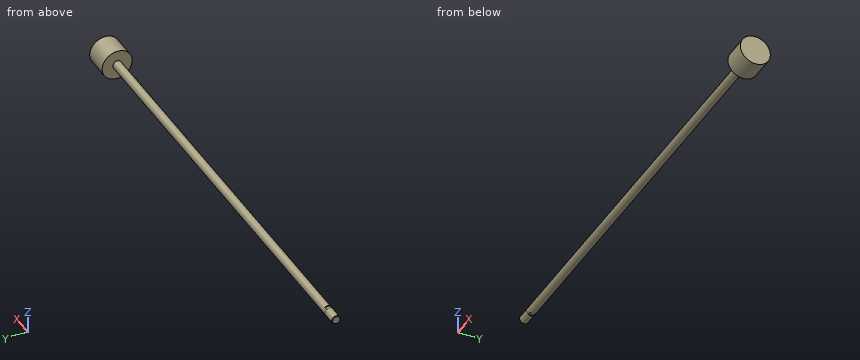
Autodesk Inventor part; units mm, degrees
ref_plane "rod_cp_XY" through (0, 0, 0) normal (1, 0, 0) x (0, 0, -1)
ref_plane "rod_cp_YZ" through (0, 0, 0) normal (0, 0, -1) x (0, 1, 0)
ref_plane "rod_cp_ZX" through (0, 0, 0) normal (0, 1, 0) x (1, 0, 0)
sketch "Sketch_1" plane through (0, 0, 0) normal (0, 0, 1) x (1, 0, 0)
  line L0 (393.5984, 0) -> (-3.175, 0)
  line L1 (-3.175, 0) -> (-3.175, 3.9624)
  line L2 (-3.175, 3.9624) -> (371.475, 3.9624)
  line L3 (371.475, 3.9624) -> (371.475, 13.5572)
  line L4 (371.475, 13.5572) -> (393.5984, 13.5572)
  line L5 (393.5984, 13.5572) -> (393.5984, 0)
  line L6 (393.5984, 0) -> (-3.175, 0)
revolve "Revolution1" add sketch "Sketch_1" angle 360 about axis through (393.5984, 0, 0) along (1, 0, 0)
sketch "Sketch_3" plane through (0, 0, 0) normal (0, 0, 1) x (1, 0, 0)
  line L0 (-3.175, 0) -> (-15.875, 0)
  line L1 (-15.875, 0) -> (-15.875, 3.3388)
  line L2 (-15.875, 3.3388) -> (-15.2451, 3.9688)
  line L3 (-15.2451, 3.9688) -> (-3.175, 3.9688)
  line L4 (-3.175, 3.9688) -> (-3.175, 0)
  line L5 (-3.175, 0) -> (-15.875, 0)
revolve "Revolution2" add sketch "Sketch_3" angle 360 about axis through (-3.175, 0, 0) along (1, 0, 0)
thread "Thread1"
sketch "Sketch_10" plane through (-3.175, 0, 0) normal (1, 0, 0) x (0, 0, -1)
  line L0 (-7.9248, 7.9248) -> (-7.9248, -7.9248)
  line L1 (-7.9248, -7.9248) -> (7.9248, -7.9248)
  line L2 (7.9248, -7.9248) -> (7.9248, 7.9248)
  line L3 (7.9248, 7.9248) -> (-7.9248, 7.9248)
  line L4 (-3.175, 3.9624) -> (-3.175, -3.9624)
  line L5 (-3.175, -3.9624) -> (3.175, -3.9624)
  line L6 (3.175, -3.9624) -> (3.175, 3.9624)
  line L7 (3.175, 3.9624) -> (-3.175, 3.9624)
extrude "Extrusion1" cut sketch "Sketch_10" along normal blind 3.175
ref_plane "rod_cp_XY" through (0, 0, 0) normal (1, 0, 0) x (0, 0, -1)
ref_plane "rod_cp_YZ" through (0, 0, 0) normal (0, 0, -1) x (0, 1, 0)
ref_plane "rod_cp_ZX" through (0, 0, 0) normal (0, 1, 0) x (1, 0, 0)
ref_plane "to_rod_clevis_XY" through (-15.875, 0, 0) normal (1, 0, 0) x (0, 0, -1)
ref_plane "to_rod_clevis_YZ" through (-15.875, 0, 0) normal (0, 0, -1) x (0, 1, 0)
ref_plane "to_rod_clevis_ZX" through (-15.875, 0, 0) normal (0, 1, 0) x (1, 0, 0)
ref_plane "rl2_XY" through (-3.175, 0, 0) normal (1, 0, 0) x (0, 0, -1)
ref_plane "rl2_YZ" through (-3.175, 0, 0) normal (0, 0, -1) x (0, 1, 0)
ref_plane "rl2_ZX" through (-3.175, 0, 0) normal (0, 1, 0) x (1, 0, 0)
ref_plane "rl1_XY" through (-15.875, 0, 0) normal (1, 0, 0) x (0, 0, -1)
ref_plane "rl1_YZ" through (-15.875, 0, 0) normal (0, 0, -1) x (0, 1, 0)
ref_plane "rl1_ZX" through (-15.875, 0, 0) normal (0, 1, 0) x (1, 0, 0)
ref_plane "thd1_XY" through (-15.875, 3.9688, 0) normal (1, 0, 0) x (0, 0, -1)
ref_plane "thd1_YZ" through (-15.875, 3.9688, 0) normal (0, 0, -1) x (0, 1, 0)
ref_plane "thd1_ZX" through (-15.875, 3.9688, 0) normal (0, 1, 0) x (1, 0, 0)
ref_plane "thd2_XY" through (-15.875, -3.9688, 0) normal (1, 0, 0) x (0, 0, -1)
ref_plane "thd2_YZ" through (-15.875, -3.9688, 0) normal (0, 0, -1) x (0, 1, 0)
ref_plane "thd2_ZX" through (-15.875, -3.9688, 0) normal (0, 1, 0) x (1, 0, 0)
ref_plane "dia1_XY" through (-3.175, 3.9624, 0) normal (1, 0, 0) x (0, 0, -1)
ref_plane "dia1_YZ" through (-3.175, 3.9624, 0) normal (0, 0, -1) x (0, 1, 0)
ref_plane "dia1_ZX" through (-3.175, 3.9624, 0) normal (0, 1, 0) x (1, 0, 0)
ref_plane "dia2_XY" through (-3.175, -3.9624, 0) normal (1, 0, 0) x (0, 0, -1)
ref_plane "dia2_YZ" through (-3.175, -3.9624, 0) normal (0, 0, -1) x (0, 1, 0)
ref_plane "dia2_ZX" through (-3.175, -3.9624, 0) normal (0, 1, 0) x (1, 0, 0)
ref_plane "wf1_XY" through (-3.175, 0, 0) normal (1, 0, 0) x (0, 0, -1)
ref_plane "wf1_YZ" through (-3.175, 0, 0) normal (0, 0, -1) x (0, 1, 0)
ref_plane "wf1_ZX" through (-3.175, 0, 0) normal (0, 1, 0) x (1, 0, 0)
ref_plane "wf2_XY" through (0, 0, 0) normal (1, 0, 0) x (0, 0, -1)
ref_plane "wf2_YZ" through (0, 0, 0) normal (0, 0, -1) x (0, 1, 0)
ref_plane "wf2_ZX" through (0, 0, 0) normal (0, 1, 0) x (1, 0, 0)
ref_plane "hh1_XY" through (421.3606, 0, 0) normal (0, 0, 1) x (1, 0, 0)
ref_plane "hh1_YZ" through (421.3606, 0, 0) normal (1, 0, 0) x (0, 1, 0)
ref_plane "hh1_ZX" through (421.3606, 0, 0) normal (0, 1, 0) x (0, 0, 1)
ref_plane "hh2_XY" through (427.7614, 0, 0) normal (0, 0, 1) x (1, 0, 0)
ref_plane "hh2_YZ" through (427.7614, 0, 0) normal (1, 0, 0) x (0, 1, 0)
ref_plane "hh2_ZX" through (427.7614, 0, 0) normal (0, 1, 0) x (0, 0, 1)
ref_plane "dia12_XY" through (0, 0, 14.1351) normal (1, 0, 0) x (0, 0, -1)
ref_plane "dia12_YZ" through (0, 0, 14.1351) normal (0, 0, -1) x (0, 1, 0)
ref_plane "dia12_ZX" through (0, 0, 14.1351) normal (0, 1, 0) x (1, 0, 0)
ref_plane "dia22_XY" through (0, 0, -14.1351) normal (1, 0, 0) x (0, 0, -1)
ref_plane "dia22_YZ" through (0, 0, -14.1351) normal (0, 0, -1) x (0, 1, 0)
ref_plane "dia22_ZX" through (0, 0, -14.1351) normal (0, 1, 0) x (1, 0, 0)
ref_plane "wfw1_XY" through (-3.175, 0, -3.175) normal (0, 1, 0) x (1, 0, 0)
ref_plane "wfw1_YZ" through (-3.175, 0, -3.175) normal (1, 0, 0) x (0, 0, -1)
ref_plane "wfw1_ZX" through (-3.175, 0, -3.175) normal (0, 0, -1) x (0, 1, 0)
ref_plane "wfw2_XY" through (-3.175, 0, 3.175) normal (0, 1, 0) x (1, 0, 0)
ref_plane "wfw2_YZ" through (-3.175, 0, 3.175) normal (1, 0, 0) x (0, 0, -1)
ref_plane "wfw2_ZX" through (-3.175, 0, 3.175) normal (0, 0, -1) x (0, 1, 0)
properties part number "0913-DX0_rod"
Geometry check sheet. Reference: the model listing, model coordinates, mm. Give positions to 0.01 mm unless a question says otherwise; leave off trailing zeros. Write each loop counter-clockwise with the first axis right and the second up, starting at its lowest first coordinate (ties: lowest second). Pieces come first, ordered by that corner, then holes.
1) Section check A-A, the plane x = 218. Record the boundary of the cut face in (y, z).
2) Section check B-B, the plane z = -7.75. Record the boundary of the cut face in (x, y) (3 decimals).
3) Material ranges on L1, parallel to X at y = 3.75, z = -4 (3 decimals); L2, parallel to Z at x = 176, y = 0.5; L3, parallel to Y at x = 345, z = 1.5, recorded low to high.
4) Gauge pin test, flat ends, axial feed: pin 1 (6 mm diameter, centred on x = 39, y = -4.5, fed in from +Z); pin 2 (2 mm diameter, centred on y = -6, z = -5.5, fed in from -X) (3 decimals); pin 3 (3.5 mm diameter, centred on x = -2, y = 0, fed in from -Z); pin 4 (0.9 mm diameter, centred on y = 0.5, z = 3.5, fed in from -X) (3 decimals). Record the tip position at first contact, or that the pin passes through.
5) Section check C-C, the plane y = -9.5. Record the boundary of the cut face in (x, z) (3 decimals), and give its area (3 significant figures).
Computed:
1. outline: circle Ø7.92 at (0, 0)
2. outline: (371.475, -11.124) - (393.598, -11.124) - (393.598, 11.124) - (371.475, 11.124) - close
3. L1: x = 371.475 to 393.598
3. L2: z = -3.93 to 3.93
3. L3: y = -3.67 to 3.67
4. pin 1: stops at z = 3.67
4. pin 2: stops at x = 371.475
4. pin 3: stops at z = -3.97
4. pin 4: stops at x = -15.875
5. outline: (371.475, -9.672) - (393.598, -9.672) - (393.598, 9.672) - (371.475, 9.672) - close
5. area: 428 mm2
